from build123d import *

# Parameters (mm, degrees)
F0_R     = 28.575
F0_R_2   = 19.4437
F1_DEPTH = 6.35
F2_SIZE  = 0.381
F3_R     = 0.254


with BuildPart() as f1:
    # F0 (on Front) → F1 (new body)
    with BuildSketch(Plane.XZ):
        Circle(F0_R)
        Circle(F0_R_2, mode=Mode.SUBTRACT)
    extrude(amount=F1_DEPTH)

    # F2
    f2_edges = [f1.edges().sort_by_distance(p)[0] for p in [
        (-19.4437, -6.35, 0),
        (-19.4437, 0, 0),
    ]]
    chamfer(f2_edges, length=F2_SIZE)

    # F3
    f3_edges = [f1.edges().sort_by_distance(p)[0] for p in [
        (-28.575, 0, 0),
        (-28.575, -6.35, 0),
    ]]
    fillet(f3_edges, radius=F3_R)


solid = f1.part
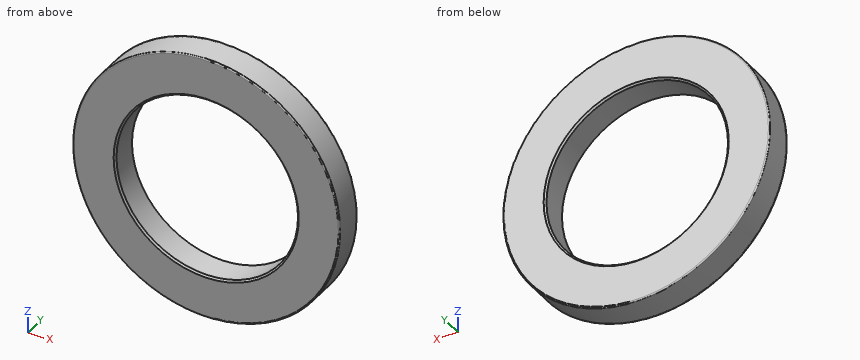
Verification items for the finished model (mm, model axes). Coordinates: 2 decimals unless noted, no trailing zeros. Order: outer loops, then holes, each group sorted by start corner. A loop starts at its lowest first (then second) coordinate and runs counter-clockwise, first axis right, second up.
1. Go/stop test with flat-tipped pins: pin 1 Ø3 at (x, z) = (-22.5, 9.5) entering from +Y; pin 2 Ø3 at (y, z) = (-1, -5.5) entering from +X. Record where each tip stops, or that it passes through.
Results found:
pin 1: stops at y = 0
pin 2: stops at x = 28.29
2. Sectioned sample at C-C, the plane y = -4.5. Record the cut outline in (x, z) (3 decimals).
Results found:
outline: circle Ø57.15 at (0, 0); hole circle Ø38.887 at (0, 0)
3. Sectioned sample at A-A, the plane z = 0. Record the cut outline in (x, y) (3 decimals), and give its area (3 significant figures).
Results found:
outline: (-28.575, -6.096) arc R0.254 ccw to (-28.321, -6.35) - (-19.825, -6.35) - (-19.444, -5.969) - (-19.444, -0.381) - (-19.825, 0) - (-28.321, 0) arc R0.254 ccw to (-28.575, -0.254) - close; (19.444, -5.969) - (19.825, -6.35) - (28.321, -6.35) arc R0.254 ccw to (28.575, -6.096) - (28.575, -0.254) arc R0.254 ccw to (28.321, 0) - (19.825, 0) - (19.444, -0.381) - close
area: 116 mm2
4. Scan lines: line 1 (Z direction, x = 0, y = -1.8) (3 decimals); line 2 (X direction, y = -2.5, z = 6.5); line 3 (Z direction, x = -17.5, y = -3.5). Record each from-to range of solid material in increasing order.
Results found:
line 1: z = -28.575 to -19.444, 19.444 to 28.575
line 2: x = -27.83 to -18.33, 18.33 to 27.83
line 3: z = -22.59 to -8.47, 8.47 to 22.59
5. Sectioned sample at B-B, the plane x = 0. Record the cut outline in (y, z) (3 decimals).
Results found:
outline: (-6.35, -28.321) arc R0.254 ccw to (-6.096, -28.575) - (-0.254, -28.575) arc R0.254 ccw to (0, -28.321) - (0, -19.825) - (-0.381, -19.444) - (-5.969, -19.444) - (-6.35, -19.825) - close; (-6.35, 19.825) - (-5.969, 19.444) - (-0.381, 19.444) - (0, 19.825) - (0, 28.321) arc R0.254 ccw to (-0.254, 28.575) - (-6.096, 28.575) arc R0.254 ccw to (-6.35, 28.321) - close
